Design review of the part built by this model. Coordinates are the model's own, in mm. A direction names the side the tool comes from. Round coordinates to 2 decimals unless told otherwise and drop trailing zeros. Loops run counter-clockwise (first coordinate to the right, second up) from the corner with the lowest first, then second, coordinate; pieces in that order, holes last. Notation, with made-up numbers: (38.5, 87.5) - (48.5, 87.5) arc R23 cw to (48.5, 122.5) - close; hole circle Ø5 at (84, 48). An arc over 180 degrees is marked (long way). Use one line per item in the form item = value. Start each with the question number.
(1) We need section A-A, the plane y = 0. Write out the cut boundary in (x, z), then the cut area to 3 significant figures.
(2) We need section C-C, the plane x = 0. Write out the cut boundary in (y, z), then the cut area to 3 significant figures.
(3) The part is to be moulded in two halves that separate along X. For faces 6 (the flat face through (40, 0, 44)), 7 (the flat face through (20, 0, 44)), 8 (the cylindrical face through (-29.86, 0.4, 77.44)), 9 (the cylindrical face through (2.08, -9.36, 12.29)), say which applies: released by +X, released by -X, zero draft, split by the parting line, or undercut.
(4) Machinability: for faces 1 (the flat face through (30, -17.5, 43)), 2 (the cylindrical face through (30.14, 0.385, 85.946)), 3 (the flat face through (-40, 0, 44)), 4 (the flat face through (-20, 0, 44)), 5 (the flat face through (30, 17.5, 43)), which of the approach directions +Z, -Z, +X, -X, +Y, -Y give a long, thin tool a straight path to every point of the face, cutting with its end or side? Answer none if there is none.
(5) We need section D-D, the plane x = -34.5. Write out the cut boundary in (y, z).
(6) Wall thickness on probe 1 along X at (y, z) = (16, 75); probe 2 along Z at (x, y) = (42.5, 44.5); probe 3 along Z at (x, y) = (28, 4.5): over which ranges is each line inside the solid? List them lowest first. Write a range as [from, to].
(7) For pin 1 (22 mm diameter, centred on x = -34, z = 53.5, fed in from -Y); pin 2 (22 mm diameter, centred on x = -26, z = 54, fed in from +Y); pin 3 (5 mm diameter, centred on x = -15, y = -13.5, fed in from +Z), all flat-tipped, find the tip position at first contact; note any pin that passes through.
(8) We need section B-B, the plane z = 21. Write out the cut boundary in (x, y), then the cut area to 3 significant figures.
from build123d import *

# Parameters (mm, degrees)
SKETCH5_R            = 9.589935832
CUT_EXTRUDE1_DEPTH   = 40
BOSS_EXTRUDE8_DEPTH  = 60
CIRPATTERN8_COUNT    = 24
SKETCH18_W           = 20
SKETCH18_H           = 35
BOSS_EXTRUDE9_DEPTH  = 50
SKETCH19_R           = 17.5
BOSS_EXTRUDE10_DEPTH = 20
SKETCH20_R           = 17.5
BOSS_EXTRUDE11_DEPTH = 20
SKETCH22_R           = 70
CUT_EXTRUDE3_DEPTH   = 65
SKETCH23_R           = 9
CUT_EXTRUDE4_DEPTH   = 90


with BuildPart() as part:
    # Sketch4 → Revolve1 (revolve)
    with BuildSketch(Plane(origin=(0, 0, 0), x_dir=(1, 0, 0), z_dir=(0, 1, 0)), mode=Mode.PRIVATE) as revolve1_sk:
        Polygon((0, 0), (0, -18.450154162), (67.865602024, -18.450154162), (67.865602024, 58.705035971), (49.02838169, 58.705035971), (49.02838169, 0), align=None)
    revolve(revolve1_sk.sketch.rotate(Axis((0, 0, -85.541623844), (0, 0, 1)), 180), axis=Axis((0, 0, -85.541623844), (0, 0, 1)))

    # Sketch5 → Cut-Extrude1 (cut)
    with BuildSketch(Plane(origin=(0, 0, 0), x_dir=(-1, 0, 0), z_dir=(0, 0, -1))):
        Circle(SKETCH5_R)
    extrude(amount=-CUT_EXTRUDE1_DEPTH, mode=Mode.SUBTRACT)

    # Sketch18 → Boss-Extrude9 (add)
    with BuildSketch(Plane.XY.offset(18.450154162)):
        with Locations((-30, 0)):
            Rectangle(SKETCH18_W, SKETCH18_H)
        with Locations((30, 0)):
            Rectangle(SKETCH18_W, SKETCH18_H)
    extrude(amount=BOSS_EXTRUDE9_DEPTH)

    # Sketch19 → Boss-Extrude10 (add)
    with BuildSketch(Plane(origin=(-20, 0, 0), x_dir=(0, 0, -1), z_dir=(1, 0, 0))):
        with Locations((-68.450154162, 0)):
            Circle(SKETCH19_R)
    extrude(amount=-BOSS_EXTRUDE10_DEPTH)

    # Sketch20 → Boss-Extrude11 (add)
    with BuildSketch(Plane(origin=(40, 0, 0), x_dir=(0, 0, -1), z_dir=(1, 0, 0))):
        with Locations((-68.450154162, 0)):
            Circle(SKETCH20_R)
    extrude(amount=-BOSS_EXTRUDE11_DEPTH)


with BuildPart() as body_2:
    # Sketch6 → Boss-Extrude8 (new body)
    with BuildSketch(Plane(origin=(0, 0, -58.705035971), x_dir=(-1, 0, 0), z_dir=(0, 0, -1))):
        Polygon((-8.362087214, 48.310016649), (-5.897089184, 44.631705328), (-3.61276171, 45.181148209), (-2.68200751, 48.954969583), align=None)
    extrude(amount=-BOSS_EXTRUDE8_DEPTH)


with BuildPart() as cirpattern8_1:
    # CirPattern8: pattern copy
    add(body_2.part.rotate(Axis((0, 0, 0), (0, 0, 1)), 1 * 360 / CIRPATTERN8_COUNT))


with BuildPart() as cirpattern8_2:
    # CirPattern8: pattern copy
    add(body_2.part.rotate(Axis((0, 0, 0), (0, 0, 1)), 2 * 360 / CIRPATTERN8_COUNT))


with BuildPart() as cirpattern8_3:
    # CirPattern8: pattern copy
    add(body_2.part.rotate(Axis((0, 0, 0), (0, 0, 1)), 3 * 360 / CIRPATTERN8_COUNT))


with BuildPart() as cirpattern8_4:
    # CirPattern8: pattern copy
    add(body_2.part.rotate(Axis((0, 0, 0), (0, 0, 1)), 4 * 360 / CIRPATTERN8_COUNT))


with BuildPart() as cirpattern8_5:
    # CirPattern8: pattern copy
    add(body_2.part.rotate(Axis((0, 0, 0), (0, 0, 1)), 5 * 360 / CIRPATTERN8_COUNT))


with BuildPart() as cirpattern8_6:
    # CirPattern8: pattern copy
    add(body_2.part.rotate(Axis((0, 0, 0), (0, 0, 1)), 6 * 360 / CIRPATTERN8_COUNT))


with BuildPart() as cirpattern8_7:
    # CirPattern8: pattern copy
    add(body_2.part.rotate(Axis((0, 0, 0), (0, 0, 1)), 7 * 360 / CIRPATTERN8_COUNT))


with BuildPart() as cirpattern8_8:
    # CirPattern8: pattern copy
    add(body_2.part.rotate(Axis((0, 0, 0), (0, 0, 1)), 8 * 360 / CIRPATTERN8_COUNT))


with BuildPart() as cirpattern8_9:
    # CirPattern8: pattern copy
    add(body_2.part.rotate(Axis((0, 0, 0), (0, 0, 1)), 9 * 360 / CIRPATTERN8_COUNT))


with BuildPart() as cirpattern8_10:
    # CirPattern8: pattern copy
    add(body_2.part.rotate(Axis((0, 0, 0), (0, 0, 1)), 10 * 360 / CIRPATTERN8_COUNT))


with BuildPart() as cirpattern8_11:
    # CirPattern8: pattern copy
    add(body_2.part.rotate(Axis((0, 0, 0), (0, 0, 1)), 11 * 360 / CIRPATTERN8_COUNT))


with BuildPart() as cirpattern8_12:
    # CirPattern8: pattern copy
    add(body_2.part.rotate(Axis((0, 0, 0), (0, 0, 1)), 12 * 360 / CIRPATTERN8_COUNT))


with BuildPart() as cirpattern8_13:
    # CirPattern8: pattern copy
    add(body_2.part.rotate(Axis((0, 0, 0), (0, 0, 1)), 13 * 360 / CIRPATTERN8_COUNT))


with BuildPart() as cirpattern8_14:
    # CirPattern8: pattern copy
    add(body_2.part.rotate(Axis((0, 0, 0), (0, 0, 1)), 14 * 360 / CIRPATTERN8_COUNT))


with BuildPart() as cirpattern8_15:
    # CirPattern8: pattern copy
    add(body_2.part.rotate(Axis((0, 0, 0), (0, 0, 1)), 15 * 360 / CIRPATTERN8_COUNT))


with BuildPart() as cirpattern8_16:
    # CirPattern8: pattern copy
    add(body_2.part.rotate(Axis((0, 0, 0), (0, 0, 1)), 16 * 360 / CIRPATTERN8_COUNT))


with BuildPart() as cirpattern8_17:
    # CirPattern8: pattern copy
    add(body_2.part.rotate(Axis((0, 0, 0), (0, 0, 1)), 17 * 360 / CIRPATTERN8_COUNT))


with BuildPart() as cirpattern8_18:
    # CirPattern8: pattern copy
    add(body_2.part.rotate(Axis((0, 0, 0), (0, 0, 1)), 18 * 360 / CIRPATTERN8_COUNT))


with BuildPart() as cirpattern8_19:
    # CirPattern8: pattern copy
    add(body_2.part.rotate(Axis((0, 0, 0), (0, 0, 1)), 19 * 360 / CIRPATTERN8_COUNT))


with BuildPart() as cirpattern8_20:
    # CirPattern8: pattern copy
    add(body_2.part.rotate(Axis((0, 0, 0), (0, 0, 1)), 20 * 360 / CIRPATTERN8_COUNT))


with BuildPart() as cirpattern8_21:
    # CirPattern8: pattern copy
    add(body_2.part.rotate(Axis((0, 0, 0), (0, 0, 1)), 21 * 360 / CIRPATTERN8_COUNT))


with BuildPart() as cirpattern8_22:
    # CirPattern8: pattern copy
    add(body_2.part.rotate(Axis((0, 0, 0), (0, 0, 1)), 22 * 360 / CIRPATTERN8_COUNT))


with BuildPart() as cirpattern8_23:
    # CirPattern8: pattern copy
    add(body_2.part.rotate(Axis((0, 0, 0), (0, 0, 1)), 23 * 360 / CIRPATTERN8_COUNT))


with BuildPart() as cut_extrude3_tool:
    # Sketch22 → Cut-Extrude3 (new body)
    with BuildSketch(Plane(origin=(0, 0, -58.705035971), x_dir=(-1, 0, 0), z_dir=(0, 0, -1))):
        Circle(SKETCH22_R)
    extrude(amount=-CUT_EXTRUDE3_DEPTH)


with BuildPart() as part_1:
    add(part.part)

    # Cut-Extrude3: cut by cut_extrude3_tool
    add(cut_extrude3_tool.part, mode=Mode.SUBTRACT)

    # Sketch23 → Cut-Extrude4 (cut)
    with BuildSketch(Plane(origin=(40, 0, 0), x_dir=(0, 0, -1), z_dir=(1, 0, 0))):
        with Locations((-68.450154162, 0)):
            Circle(SKETCH23_R)
    extrude(amount=-CUT_EXTRUDE4_DEPTH, mode=Mode.SUBTRACT)


with BuildPart() as body_2_1:
    add(body_2.part)

    # Cut-Extrude3: cut by cut_extrude3_tool
    add(cut_extrude3_tool.part, mode=Mode.SUBTRACT)


with BuildPart() as cirpattern8_1_1:
    add(cirpattern8_1.part)

    # Cut-Extrude3: cut by cut_extrude3_tool
    add(cut_extrude3_tool.part, mode=Mode.SUBTRACT)


with BuildPart() as cirpattern8_2_1:
    add(cirpattern8_2.part)

    # Cut-Extrude3: cut by cut_extrude3_tool
    add(cut_extrude3_tool.part, mode=Mode.SUBTRACT)


with BuildPart() as cirpattern8_3_1:
    add(cirpattern8_3.part)

    # Cut-Extrude3: cut by cut_extrude3_tool
    add(cut_extrude3_tool.part, mode=Mode.SUBTRACT)


with BuildPart() as cirpattern8_4_1:
    add(cirpattern8_4.part)

    # Cut-Extrude3: cut by cut_extrude3_tool
    add(cut_extrude3_tool.part, mode=Mode.SUBTRACT)


with BuildPart() as cirpattern8_5_1:
    add(cirpattern8_5.part)

    # Cut-Extrude3: cut by cut_extrude3_tool
    add(cut_extrude3_tool.part, mode=Mode.SUBTRACT)


with BuildPart() as cirpattern8_6_1:
    add(cirpattern8_6.part)

    # Cut-Extrude3: cut by cut_extrude3_tool
    add(cut_extrude3_tool.part, mode=Mode.SUBTRACT)


with BuildPart() as cirpattern8_7_1:
    add(cirpattern8_7.part)

    # Cut-Extrude3: cut by cut_extrude3_tool
    add(cut_extrude3_tool.part, mode=Mode.SUBTRACT)


with BuildPart() as cirpattern8_8_1:
    add(cirpattern8_8.part)

    # Cut-Extrude3: cut by cut_extrude3_tool
    add(cut_extrude3_tool.part, mode=Mode.SUBTRACT)


with BuildPart() as cirpattern8_9_1:
    add(cirpattern8_9.part)

    # Cut-Extrude3: cut by cut_extrude3_tool
    add(cut_extrude3_tool.part, mode=Mode.SUBTRACT)


with BuildPart() as cirpattern8_10_1:
    add(cirpattern8_10.part)

    # Cut-Extrude3: cut by cut_extrude3_tool
    add(cut_extrude3_tool.part, mode=Mode.SUBTRACT)


with BuildPart() as cirpattern8_11_1:
    add(cirpattern8_11.part)

    # Cut-Extrude3: cut by cut_extrude3_tool
    add(cut_extrude3_tool.part, mode=Mode.SUBTRACT)


with BuildPart() as cirpattern8_12_1:
    add(cirpattern8_12.part)

    # Cut-Extrude3: cut by cut_extrude3_tool
    add(cut_extrude3_tool.part, mode=Mode.SUBTRACT)


with BuildPart() as cirpattern8_13_1:
    add(cirpattern8_13.part)

    # Cut-Extrude3: cut by cut_extrude3_tool
    add(cut_extrude3_tool.part, mode=Mode.SUBTRACT)


with BuildPart() as cirpattern8_14_1:
    add(cirpattern8_14.part)

    # Cut-Extrude3: cut by cut_extrude3_tool
    add(cut_extrude3_tool.part, mode=Mode.SUBTRACT)


with BuildPart() as cirpattern8_15_1:
    add(cirpattern8_15.part)

    # Cut-Extrude3: cut by cut_extrude3_tool
    add(cut_extrude3_tool.part, mode=Mode.SUBTRACT)


with BuildPart() as cirpattern8_16_1:
    add(cirpattern8_16.part)

    # Cut-Extrude3: cut by cut_extrude3_tool
    add(cut_extrude3_tool.part, mode=Mode.SUBTRACT)


with BuildPart() as cirpattern8_17_1:
    add(cirpattern8_17.part)

    # Cut-Extrude3: cut by cut_extrude3_tool
    add(cut_extrude3_tool.part, mode=Mode.SUBTRACT)


with BuildPart() as cirpattern8_18_1:
    add(cirpattern8_18.part)

    # Cut-Extrude3: cut by cut_extrude3_tool
    add(cut_extrude3_tool.part, mode=Mode.SUBTRACT)


with BuildPart() as cirpattern8_19_1:
    add(cirpattern8_19.part)

    # Cut-Extrude3: cut by cut_extrude3_tool
    add(cut_extrude3_tool.part, mode=Mode.SUBTRACT)


with BuildPart() as cirpattern8_20_1:
    add(cirpattern8_20.part)

    # Cut-Extrude3: cut by cut_extrude3_tool
    add(cut_extrude3_tool.part, mode=Mode.SUBTRACT)


with BuildPart() as cirpattern8_21_1:
    add(cirpattern8_21.part)

    # Cut-Extrude3: cut by cut_extrude3_tool
    add(cut_extrude3_tool.part, mode=Mode.SUBTRACT)


with BuildPart() as cirpattern8_22_1:
    add(cirpattern8_22.part)

    # Cut-Extrude3: cut by cut_extrude3_tool
    add(cut_extrude3_tool.part, mode=Mode.SUBTRACT)


with BuildPart() as cirpattern8_23_1:
    add(cirpattern8_23.part)

    # Cut-Extrude3: cut by cut_extrude3_tool
    add(cut_extrude3_tool.part, mode=Mode.SUBTRACT)


solid = part_1.part
Data:
q1.outline = (-67.87, 6.29) - (-9.59, 6.29) - (-9.59, 18.45) - (-20, 18.45) - (-20, 59.45) - (-40, 59.45) - (-40, 18.45) - (-67.87, 18.45) - close; (-40, 77.45) - (-20, 77.45) - (-20, 85.95) - (-40, 85.95) - close; (9.59, 6.29) - (67.87, 6.29) - (67.87, 18.45) - (40, 18.45) - (40, 59.45) - (20, 59.45) - (20, 18.45) - (9.59, 18.45) - close; (20, 77.45) - (40, 77.45) - (40, 85.95) - (20, 85.95) - close
q1.area = 3,400 mm^2
q2.outline = (-67.87, 6.29) - (-9.59, 6.29) - (-9.59, 18.45) - (-67.87, 18.45) - close; (9.59, 6.29) - (67.87, 6.29) - (67.87, 18.45) - (9.59, 18.45) - close
q2.area = 1,420 mm^2
q3.face_6 = released by +X
q3.face_7 = undercut
q3.face_8 = zero draft
q3.face_9 = undercut
q4.face_1 = +Z, +X, -X, -Y
q4.face_2 = +Z, +X, -X
q4.face_3 = +Z, -X, +Y, -Y
q4.face_4 = +Z, +Y, -Y
q4.face_5 = +Z, +X, -X, +Y
q5.outline = (-58.44, 6.29) - (58.44, 6.29) - (58.44, 18.45) - (17.5, 18.45) - (17.5, 68.45) arc R17.5 ccw to (-17.5, 68.45) - (-17.5, 18.45) - (-58.44, 18.45) - close; hole circle Ø18 at (0, 68.45)
q6.probe_1 = [-40, -20], [20, 40]
q6.probe_2 = [6.29, 18.45]
q6.probe_3 = [6.29, 60.66], [76.24, 85.36]
q7.pin_1 = -17.5
q7.pin_2 = 17.5
q7.pin_3 = 18.45
q8.outline = (-40, -17.5) - (-20, -17.5) - (-20, 17.5) - (-40, 17.5) - close; (20, -17.5) - (40, -17.5) - (40, 17.5) - (20, 17.5) - close
q8.area = 1,400 mm^2
